```python
from build123d import *

# Parameters (mm, degrees)
SKETCH1_W           = 40
SKETCH1_H           = 30
BOSS_EXTRUDE1_DEPTH = 4
SKETCH4_W           = 28
SKETCH4_H           = 14
CUT_EXTRUDE1_DEPTH  = 5.5
SKETCH5_W           = 40
SKETCH5_H           = 5.5
BOSS_EXTRUDE2_DEPTH = 15
SKETCH6_R           = 1.65
CUT_EXTRUDE3_DEPTH  = 15
RIB1_REACH          = 50.297
SKETCH8_WALL_W      = 127.321837908
SKETCH8_WALL_H      = 2
RIB14_START         = -2
RIB14_DEPTH         = 2
FILLET1_R           = 1


# Read off the part's stored shape, not the designer's step: Rib14
with BuildPart() as part:
    # Sketch1 → Boss-Extrude1 (new body)
    with BuildSketch(Plane.XY):
        with Locations((-0.222222222, -4.277777778)):
            Rectangle(SKETCH1_W, SKETCH1_H)
    extrude(amount=BOSS_EXTRUDE1_DEPTH)

    # Sketch4 → Cut-Extrude1 (cut)
    with BuildSketch(Plane.XY.offset(4)):
        with Locations((-0.222222222, -1.777777778)):
            Rectangle(SKETCH4_W, SKETCH4_H)
    extrude(amount=-CUT_EXTRUDE1_DEPTH, mode=Mode.SUBTRACT)

    # Sketch5 → Boss-Extrude2 (add)
    with BuildSketch(Plane.XY.offset(4)):
        with Locations((-0.222222222, -16.527777778)):
            Rectangle(SKETCH5_W, SKETCH5_H)
    extrude(amount=BOSS_EXTRUDE2_DEPTH)

    # Sketch6 → Cut-Extrude3 (cut)
    with BuildSketch(Plane.XZ.offset(19.277777778)):
        with Locations(Location((-12.222222222, 13, 0), (0, 0, 270))):
            Circle(SKETCH6_R)
        with Locations(Location((-0.222222222, 13, 0), (0, 0, 270))):
            Circle(SKETCH6_R)
        with Locations(Location((11.777777778, 13, 0), (0, 0, 270))):
            Circle(SKETCH6_R)
    extrude(amount=-CUT_EXTRUDE3_DEPTH, mode=Mode.SUBTRACT)

    # Sketch8 wall → Rib1 (add, up to next)
    with BuildSketch(Plane(origin=(-20.222222222, -1.527777778, 11.5), x_dir=(0, -0.852851304076, 0.522153859639), z_dir=(0, 0.522153859639, 0.852851304076)), mode=Mode.PRIVATE) as rib1_sk1:
        with Locations((0, 1)):
            Rectangle(SKETCH8_WALL_W, SKETCH8_WALL_H)
    rib1_tool1 = extrude(rib1_sk1.sketch, amount=-RIB1_REACH, mode=Mode.PRIVATE) - part.part
    add(rib1_tool1.solids().sort_by_distance((-20.222222222, -1.527777778, 11.5))[0])

    # Rib14 outline → Rib14 (add)
    with BuildSketch(Plane(origin=(19.777777778, 0, 0), x_dir=(0, 0, -1), z_dir=(1, 0, 0)).offset(RIB14_START)):
        Polygon((-4, 10.722222222), (-19, -13.777777778), (-4, -13.777777778), align=None)
    extrude(amount=RIB14_DEPTH)

    # Fillet1
    fillet1_edges = [part.edges().sort_by_distance(p)[0] for p in [
        (-18.222222222, -1.527777778, 4),
        (-18.222222222, -13.777777778, 11.5),
        (-0.222222222, -13.777777778, 4),
        (17.777777778, -1.527777778, 4),
        (17.777777778, -13.777777778, 11.5),
    ]]
    fillet(fillet1_edges, radius=FILLET1_R)


solid = part.part
```
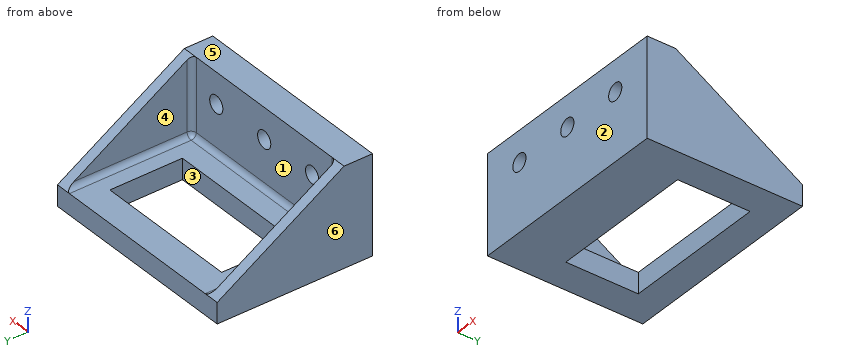
Input: part model. Units: mm. Frame: model coordinates. Face numbers are marked on the shaded views. A direction names the side the tool comes from. Give positions to 0.01 mm unless a question says otherwise; leave off trailing zeros. Order: outer loops, then holes, each group sorted by start corner. A loop starts at its lowest first (then second) coordinate and runs counter-clockwise, first axis right, second up.
1. Cut plane C-C (y = -1.5). Return loops of the section in (x, z).
Computed:
outline: (-20.22, 0) - (-14.22, 0) - (-14.22, 4) - (-17.22, 4) arc R1 cw to (-18.22, 5) - (-18.22, 11.48) - (-20.22, 11.48) - close; (13.78, 0) - (19.78, 0) - (19.78, 11.48) - (17.78, 11.48) - (17.78, 5) arc R1 cw to (16.78, 4) - (13.78, 4) - close
2. Pin query (flat end, axial travel): pin 1 Ø12 at (x, y) = (8, -1) entering from +Z; pin 2 Ø4 at (x, z) = (-0.22, 13) entering from +Y. Return the tip coordinate at first contact, or that it passes through.
Computed:
pin 1: stops at z = 4
pin 2: stops at y = -13.78
3. Draft query along X for the marked faces 4, 5 and 6. Return one class per face: released by +X, released by -X, zero draft, split by the parting line, or undercut.
Computed:
face 4: undercut
face 5: zero draft
face 6: released by -X
4. Cut plane D-D (x = 12.5). Return loops of the section in (y, z), and give its area (3 significant figures).
Computed:
outline: (-19.28, 0) - (-8.78, 0) - (-8.78, 4) - (-12.78, 4) arc R1 cw to (-13.78, 5) - (-13.78, 11.52) - (-19.28, 11.52) - close; (-19.28, 14.48) - (-13.78, 14.48) - (-13.78, 19) - (-19.28, 19) - close; (5.22, 0) - (10.72, 0) - (10.72, 4) - (5.22, 4) - close
area: 130 mm2
5. Line query: probe 1 along X at (y, z) = (-17.2, 13); probe 2 along X at (y, z) = (-5, 5); probe 3 along X at (y, z) = (-1.5, 3.25). Output: solid intervals per line, ascending.
Computed:
probe 1: x = -20.22 to -13.87, -10.57 to -1.87, 1.43 to 10.13, 13.43 to 19.78
probe 2: x = -20.22 to -18.22, 17.78 to 19.78
probe 3: x = -20.22 to -14.22, 13.78 to 19.78
6. Cut plane B-B (z = 13). Return loops of the section in (x, y).
Computed:
outline: (-20.22, -19.28) - (-13.87, -19.28) - (-13.87, -13.78) - (-17.22, -13.78) arc R1 cw to (-18.22, -12.78) - (-18.22, -3.98) - (-20.22, -3.98) - close; (-10.57, -19.28) - (-1.87, -19.28) - (-1.87, -13.78) - (-10.57, -13.78) - close; (1.43, -19.28) - (10.13, -19.28) - (10.13, -13.78) - (1.43, -13.78) - close; (13.43, -19.28) - (19.78, -19.28) - (19.78, -3.98) - (17.78, -3.98) - (17.78, -12.78) arc R1 cw to (16.78, -13.78) - (13.43, -13.78) - close
7. Set-up query: the marked faces 1, 2 and 3. Return all of +Z, -Z, +X, -X, +Y, -Y with unobstructed straight access to the full face (end or side cutting, diameter ignored); none if empty.
Computed:
face 1: +Z, +Y
face 2: +Z, -Z, +X, -X, -Y
face 3: +Z, -Z
8. Cut plane A-A (x = 7). Return loops of the section in (y, z).
Computed:
outline: (-19.28, 0) - (-8.78, 0) - (-8.78, 4) - (-12.78, 4) arc R1 cw to (-13.78, 5) - (-13.78, 19) - (-19.28, 19) - close; (5.22, 0) - (10.72, 0) - (10.72, 4) - (5.22, 4) - close
